CAD build for the part. Positions are in the model's coordinates, mm. A direction names the side the tool comes from. Round coordinates to 2 decimals unless told otherwise and drop trailing zeros. Loops run counter-clockwise (first coordinate to the right, second up) from the corner with the lowest first, then second, coordinate; pieces in that order, holes last. Notation, with made-up numbers: (87.25, -20) - (130.25, -20) arc R28 ccw to (130.25, 10) - close; hole circle Ø4 at (-14.75, -7.75). An arc over 180 degrees is marked (long way). One line per question, with ' | ' between items.
```python
from build123d import *

# Parameters (mm, degrees)
SKETCH2_W             = 50
SKETCH2_H             = 50
SKETCH2_W_2           = 36.05
SKETCH2_H_2           = 36.05
BOSS_EXTRUDE2_DEPTH   = 5
SKETCH1_W             = 50
SKETCH1_H             = 50
SKETCH1_W_2           = 40.05
SKETCH1_H_2           = 40.05
BOSS_EXTRUDE4_DEPTH   = 40
BOSS_EXTRUDE5_START   = -25
BOSS_EXTRUDE5_DEPTH   = 50
BOSS_EXTRUDE5_2_DEPTH = 4.975
BOSS_EXTRUDE5_START_2 = 20.025
BOSS_EXTRUDE5_3_DEPTH = 4.975
SKETCH7_W             = 50.771330761
SKETCH7_H             = 7
BOSS_EXTRUDE6_DEPTH   = 5
SKETCH8_R             = 1.6
CUT_EXTRUDE1_DEPTH    = 5


# Read off the part's stored shape, not the designer's step: Boss-Extrude5
with BuildPart() as part:
    # Sketch2 → Boss-Extrude2 (new body)
    with BuildSketch(Plane(origin=(0, 0, 0), x_dir=(1, 0, 0), z_dir=(0, 1, 0))):
        Rectangle(SKETCH2_W, SKETCH2_H)
        Rectangle(SKETCH2_W_2, SKETCH2_H_2, mode=Mode.SUBTRACT)
    extrude(amount=BOSS_EXTRUDE2_DEPTH)

    # Sketch1 → Boss-Extrude4 (add)
    with BuildSketch(Plane(origin=(0, 0, 0), x_dir=(1, 0, 0), z_dir=(0, 1, 0))):
        Rectangle(SKETCH1_W, SKETCH1_H)
        Rectangle(SKETCH1_W_2, SKETCH1_H_2, mode=Mode.SUBTRACT)
    extrude(amount=BOSS_EXTRUDE4_DEPTH)

    # Boss-Extrude5 outline → Boss-Extrude5 (add)
    with BuildSketch(Plane.XY.offset(BOSS_EXTRUDE5_START)):
        Polygon((25, 40), (25, 48.81635), (20.025, 47.939123175), (20.025, 40), align=None)
        Polygon((-20.025, 40), (-20.025, 40.877226825), (-25, 40), align=None)
    extrude(amount=BOSS_EXTRUDE5_DEPTH)

    # Boss-Extrude5 2 outline → Boss-Extrude5 2 (add)
    with BuildSketch(Plane.XY.offset(BOSS_EXTRUDE5_START)):
        Polygon((20.025, 40), (20.025, 47.939123175), (-20.025, 40.877226825), (-20.025, 40), align=None)
    extrude(amount=BOSS_EXTRUDE5_2_DEPTH)

    # Boss-Extrude5 3 outline → Boss-Extrude5 3 (add)
    with BuildSketch(Plane.XY.offset(BOSS_EXTRUDE5_START_2)):
        Polygon((20.025, 40), (20.025, 47.939123175), (-20.025, 40.877226825), (-20.025, 40), align=None)
    extrude(amount=BOSS_EXTRUDE5_3_DEPTH)

    # Sketch7 → Boss-Extrude6 (add)
    with BuildSketch(Plane(origin=(-7.59424597, 43.069104391, 0), x_dir=(0.984807749763281, 0.17364819609251012, 0), z_dir=(-0.17364819609251012, 0.984807749763281, 0))):
        with Locations((7.71139948, 28.5)):
            Rectangle(SKETCH7_W, SKETCH7_H)
        with Locations((7.71139948, -28.5)):
            Rectangle(SKETCH7_W, SKETCH7_H)
    extrude(amount=-BOSS_EXTRUDE6_DEPTH)

    # Sketch8 → Cut-Extrude1 (cut)
    with BuildSketch(Plane(origin=(-7.59424597, 43.069104391, 0), x_dir=(0.984807749763281, 0.17364819609251012, 0), z_dir=(-0.17364819609251012, 0.984807749763281, 0))):
        with Locations(Location((-14.1742659, -28.5, 0), (0, 0, 180))):
            Circle(SKETCH8_R)
        with Locations((29.597064861, -28.5)):
            Circle(SKETCH8_R)
        with Locations(Location((29.597064861, 28.5, 0), (0, 0, 180))):
            Circle(SKETCH8_R)
        with Locations((-14.1742659, 28.5)):
            Circle(SKETCH8_R)
    extrude(amount=-CUT_EXTRUDE1_DEPTH, mode=Mode.SUBTRACT)


solid = part.part
```
(1) Cut at A-A, the plane z = -6.5. Write the cut outline in (x, y) (3 decimals).
Results found:
outline: (-25, 0) - (-18.025, 0) - (-18.025, 5) - (-20.025, 5) - (-20.025, 40.877) - (-25, 40) - close; (18.025, 0) - (25, 0) - (25, 48.816) - (20.025, 47.939) - (20.025, 5) - (18.025, 5) - close
(2) Drop flat-ended pins along their axis: P1, Ø6, axis at x = -10, z = 18, coming from the +Y side; P2, Ø1.5, axis at y = 2, z = 4.5, coming from the +X side; P3, Ø12, axis at x = -18.5, y = 21.5, coming from the +Z side; P4, Ø1, axis at x = 25.5, y = 47.5, coming from the +Z side. Give the stop position or say it passes through.
Results found:
P1: stops at y = 43.04 | P2: stops at x = 25 | P3: stops at z = 25 | P4: stops at z = 32
(3) Cut at D-D, the plane z = 19. Write the cut outline in (x, y) (3 decimals).
Results found:
outline: (-25, 0) - (25, 0) - (25, 48.816) - (20.025, 47.939) - (20.025, 5) - (-20.025, 5) - (-20.025, 40.877) - (-25, 40) - close
(4) Cut at C-C, the plane x = 0. Write the cut outline in (y, z) (3 decimals).
Results found:
outline: (0, -25) - (39.331, -25) - (39.331, -32) - (44.408, -32) - (44.408, -20.025) - (5, -20.025) - (5, -18.025) - (0, -18.025) - close; (0, 18.025) - (5, 18.025) - (5, 20.025) - (44.408, 20.025) - (44.408, 32) - (39.331, 32) - (39.331, 25) - (0, 25) - close
(5) Two-plate mould, pull along Z, no slides. Class faces 1 (the face through (-25, 20, 0)), 2 (the face through (0, 22, -25)), 3 (the face through (0, 2, 18.025)), 4 (the face through (0, 27, -20.025)): released by +Z, released by -Z, zero draft, split by the parting line, or undercut.
Results found:
face 1: zero draft | face 2: released by -Z | face 3: undercut | face 4: undercut
(6) Cut at B-B, the plane y = 12.5. Write the cut outline in (x, z) (3 decimals), then the cut area to 3 significant figures.
Results found:
outline: (-25, -25) - (25, -25) - (25, 25) - (-25, 25) - close; hole (-20.025, -20.025) - (20.025, -20.025) - (20.025, 20.025) - (-20.025, 20.025) - close | area: 896 mm²
(7) Tool access for faces 5 (the face through (-24.57, 37.57, -28.45)), 6 (the face through (0.518, 39.422, -28.549)), 7 (the face through (0, 2, -18.025)): list every direction of +Z, -Z, +X, -X, +Y, -Y with a clear straight run to the whole face (end or side of a thin tool).
Results found:
face 5: -Z, -X, -Y | face 6: -Z, +X, -Y | face 7: +Y, -Y
(8) Probe L1, parallel to X at y = 15.5, z = -12 (3 decimals); L2, parallel to Z at x = -3, y = 41 (3 decimals). List the from-to ranges inside material, lowest first.
Results found:
L1: x = -25 to -20.025, 20.025 to 25 | L2: z = -32 to -20.025, 20.025 to 32
